Geometry: final body of the model. Coordinates: model frame, mm. A direction names the side the tool comes from. Give positions to 0.01 mm unless a question says otherwise; leave off trailing zeros. Write each loop counter-clockwise with the first axis right and the second up, starting at its lowest first coordinate (ties: lowest second). Pieces come first, ordered by that corner, then holes. Notation, with made-up numbers: M -1,58.25 L 58,58.25 A21 ccw 58,76.25 Z; hole C 27.5,44 d7. An arc over 180 degrees is marked long. Use a Markdown table: item, result. Add a question column.
(1) Pin query (flat end, axial travel): pin 1 Ø2.5 at (x, y) = (3.5, 4) entering from -Z; pin 2 Ø1.6 at (x, y) = (-4.5, 3.5) entering from -Z; pin 3 Ø5 at (x, y) = (-2.5, 4.5) entering from +Z; pin 4 Ø1.1 at (x, z) = (0.5, 4) entering from -Y. Return the tip coordinate at first contact, or that it passes through.
(2) Material intervals for L1, parallel to Y at x = 0, z = 1.65 (3 decimals); L2, parallel to X at y = 6.75, z = 2.05; L3, parallel to Y at x = -2.25, z = 2.4, sorted ascending.
(3) Cut plane C-C (y = 1). Output: boundary loops of the cut face in (x, z), plus the area to 3 significant figures.
(4) Reachability of faces 1 (the flat face through (-1.75, 0, 4)), 2 (the flat face through (0, 1, 0)) from +Z, -Z, +X, -X, +Y, -Y: full face, straight path, thin tool, end or side. Return the list, or none.
(5) Cut plane D-D (z = 1.95). Output: boundary loops of the cut face in (x, y) (3 decimals), plus the area to 3 significant figures.
(6) Cut plane A-A (x = 6.75). Output: boundary loops of the cut face in (y, z).
(7) Draft query along Y for faces 3 (the cylindrical face through (9.06, 7.71, 1.73)), 4 (the flat face through (1.75, 0, 4)). Return one class per face: released by +Y, released by -Y, zero draft, split by the parting line, or undercut.
Autodesk Fusion 360 part; units mm, degrees
sketch "Sketch1" plane through (0, 0, 0) normal (0, 0, 1) x (1, 0, 0)
  line L0 (-3, 10.6) -> (3, 10.6) construction
  line L1 (3, 10.6) -> (3, 4.6) construction
  line L2 (3, 4.6) -> (-3, 4.6) construction
  line L3 (-3, 4.6) -> (-3, 10.6) construction
  line L4 (0, -7.6) -> (0, 7.6) construction
  line L5 (0, 0) -> (-6, 0) construction
  line L6 (-3, 10.6) -> (3, 4.6) construction
  line L7 (3, 10.6) -> (-3, 4.6) construction
  line L8 (-3, -4.6) -> (3, -4.6) construction
  line L9 (3, -4.6) -> (3, -10.6) construction
  line L10 (3, -10.6) -> (-3, -10.6) construction
  line L11 (-3, -10.6) -> (-3, -4.6) construction
  line L12 (4.6, 3) -> (10.6, 3) construction
  line L13 (10.6, 3) -> (10.6, -3) construction
  line L14 (10.6, -3) -> (4.6, -3) construction
  line L15 (4.6, -3) -> (4.6, 3) construction
  line L16 (-10.6, 3) -> (-4.6, 3) construction
  line L17 (-4.6, 3) -> (-4.6, -3) construction
  line L18 (-4.6, -3) -> (-10.6, -3) construction
  line L19 (-10.6, -3) -> (-10.6, 3) construction
  line L20 (-7.6, 0) -> (7.6, 0) construction
  line L21 (-10.6, 3) -> (-4.6, -3) construction
  line L22 (-4.6, 3) -> (-10.6, -3) construction
  line L23 (-3, -10.6) -> (3, -4.6) construction
  line L24 (-3, -4.6) -> (3, -10.6) construction
  line L25 (4.6, 3) -> (10.6, -3) construction
  line L26 (10.6, 3) -> (4.6, -3) construction
  dimension "d1" = 6
  dimension "d3" = 15.2
sketch "Sketch5" plane through (0, 0, 0) normal (0, 0, 1) x (1, 0, 0)
  line L0 (-3.5, 3.5) -> (3.5, 3.5)
  line L1 (3.5, 3.5) -> (3.5, -3.5)
  line L2 (3.5, -3.5) -> (-3.5, -3.5)
  line L3 (-3.5, -3.5) -> (-3.5, 3.5)
  line L4 (-3.5, 3.5) -> (3.5, -3.5) construction
  line L5 (3.5, 3.5) -> (-3.5, -3.5) construction
  dimension "d11" = 7
extrude "Extrude4" add sketch "Sketch5" along normal blind 3.5 makes body 1
sketch "Sketch6" plane through (0, 0, 0) normal (0, 0, 1) x (1, 0, 0)
  circle A0 centre (-6.75, 6.75) radius 2.5
  circle A1 centre (6.75, 6.75) radius 2.5
  circle A2 centre (6.75, -6.75) radius 2.5
  circle A3 centre (-6.75, -6.75) radius 2.5
  line L0 (-6.75, 6.75) -> (6.75, 6.75) construction
  line L1 (6.75, 6.75) -> (6.75, -6.75) construction
  line L2 (6.75, -6.75) -> (-6.75, -6.75) construction
  line L3 (-6.75, -6.75) -> (-6.75, 6.75) construction
  line L4 (6.75, 6.75) -> (-6.75, -6.75) construction
  line L5 (-6.75, 6.75) -> (6.75, -6.75) construction
  point P0 (-7.6, 0)
  point P1 (7.6, 0)
  point P2 (0, 7.6)
  point P3 (0, -7.6)
  dimension "d14" = 5
  dimension "d15" = 13.5
extrude "Extrude5" add sketch "Sketch6" along normal blind 3.5 separate body makes body 2 at (9.2376, 6.5011, 2.3333) makes body 3 at (9.2376, -6.9989, 2.3333) makes body 4 at (-4.2624, 6.5011, 2.3333) makes body 5 at (-4.2624, -6.9989, 2.3333)
ref_plane "WorkPlane1" through (0, 0, 0.75) normal (0, 0, 1) x (1, 0, 0)
sketch "Sketch7" plane through (0, 0, 0.75) normal (0, 0, 1) x (1, 0, 0)
  line L0 (-5.594, 4.5333) -> (4.5333, -5.594)
  line L1 (4.5333, -5.594) -> (5.594, -4.5333)
  line L2 (5.594, -4.5333) -> (-4.5333, 5.594)
  line L3 (-4.5333, 5.594) -> (-5.594, 4.5333)
  line L4 (5.594, 4.5333) -> (4.5333, 5.594)
  line L5 (4.5333, 5.594) -> (-5.594, -4.5333)
  line L6 (-5.594, -4.5333) -> (-4.5333, -5.594)
  line L7 (-4.5333, -5.594) -> (5.594, 4.5333)
  line L8 (-7.6, 0) -> (7.6, 0)
  line L9 (-1.0607, 0) -> (1.0607, 0) construction
  line L10 (0, -7.6) -> (0, 7.6) construction
  circle A0 centre (6.75, 6.75) radius 2.5 construction
  circle A1 centre (-6.75, 6.75) radius 2.5 construction
  circle A2 centre (-6.75, -6.75) radius 2.5 construction
  circle A3 centre (6.75, -6.75) radius 2.5 construction
  dimension "d18" = 45
  dimension "d19" = 1.5
extrude "Extrude6" add sketch "Sketch7" along normal up to surface (2.75 mm away) contours L0 L2 L3 L5 | L0 L5 L6 L7 | L0 L1 L2 L7 | L2 L4 L5 L7 bodies 1 2 3 4 5
sketch "Sketch9" plane through (0, 0, 0) normal (0, 0, 1) x (1, 0, 0)
  circle A0 centre (0, 0) radius 0.675
  dimension "d23" = 1.35
extrude "Extrude7" cut sketch "Sketch9" along normal blind 3 bodies 1
sketch "Sketch10" plane through (0, 0, 3.5) normal (0, 0, 1) x (-1, 0, 0)
  arc A0 (4.5333, -5.594) -> (5.594, -4.5333) centre (6.75, -6.75) ccw
  line L0 (5.594, -4.5333) -> (3.5, -2.4393)
  line L1 (3.5, -2.4393) -> (3.5, 2.4393)
  line L2 (3.5, 2.4393) -> (5.594, 4.5333)
  arc A1 (5.594, 4.5333) -> (4.5333, 5.594) centre (6.75, 6.75) ccw
  line L3 (4.5333, 5.594) -> (2.4393, 3.5)
  line L4 (2.4393, 3.5) -> (-2.4393, 3.5)
  line L5 (-2.4393, 3.5) -> (-4.5333, 5.594)
  arc A2 (-4.5333, 5.594) -> (-5.594, 4.5333) centre (-6.75, 6.75) ccw
  line L6 (-5.594, 4.5333) -> (-3.5, 2.4393)
  line L7 (-3.5, 2.4393) -> (-3.5, -2.4393)
  line L8 (-3.5, -2.4393) -> (-5.594, -4.5333)
  arc A3 (-5.594, -4.5333) -> (-4.5333, -5.594) centre (-6.75, -6.75) ccw
  line L9 (-4.5333, -5.594) -> (-2.4393, -3.5)
  line L10 (-2.4393, -3.5) -> (2.4393, -3.5)
  line L11 (2.4393, -3.5) -> (4.5333, -5.594)
  line L12 (1.75, -1.25) -> (-1.75, -1.25)
  line L13 (-1.75, -1.25) -> (-1.75, 1.25)
  line L14 (-1.75, 1.25) -> (1.75, 1.25)
  line L15 (1.75, 1.25) -> (1.75, -1.25)
  line L16 (1.75, -1.25) -> (-1.75, 1.25) construction
  line L17 (-1.75, -1.25) -> (1.75, 1.25) construction
  dimension "d26" = 3.5
  dimension "d27" = 2.5
extrude "Extrude8" add sketch "Sketch10" along normal blind 1 contours L12 L13 L14 L15 bodies 1
Answer list:
| question | item | result |
|---|---|---|
| 1 | pin 1 | z = 0 |
| 1 | pin 2 | z = 0.75 |
| 1 | pin 3 | z = 3.5 |
| 1 | pin 4 | y = -3.5 |
| 2 | L1 | -3.5 to -0.675, 0.675 to 3.5 |
| 2 | L2 | -9.25 to -4.25, 4.25 to 9.25 |
| 2 | L3 | -3.5 to 3.5 |
| 3 | outline | M -3.5,0 L 3.5,0 L 3.5,3.5 L 1.75,3.5 L 1.75,4.5 L -1.75,4.5 L -1.75,3.5 L -3.5,3.5 Z |
| 3 | area | 28.0 mm² |
| 4 | face 1 | +Z, -X, +Y, -Y |
| 4 | face 2 | -Z, +X, -X, +Y, -Y |
| 5 | outline | M -5.594,-4.533 A2.5 ccw long -4.533,-5.594 L -2.439,-3.5 L 2.439,-3.5 L 4.533,-5.594 A2.5 ccw long 5.594,-4.533 L 3.5,-2.439 L 3.5,2.439 L 5.594,4.533 A2.5 ccw long 4.533,5.594 L 2.439,3.5 L -2.439,3.5 L -4.533,5.594 A2.5 ccw long -5.594,4.533 L -3.5,2.439 L -3.5,-2.439 Z; hole C 0,0 d1.35 |
| 5 | area | 141 mm² |
| 6 | outline | M -9.25,0 L -4.25,0 L -4.25,3.5 L -9.25,3.5 Z; M 4.25,0 L 9.25,0 L 9.25,3.5 L 4.25,3.5 Z |
| 7 | face 3 | undercut |
| 7 | face 4 | zero draft |
